Source: CAD feature listing. Evaluate the final solid. Frame: model axes, mm. Give positions to 0.01 mm unless a question says otherwise; leave off trailing zeros. Write each loop counter-clockwise with the first axis right and the second up, starting at its lowest first coordinate (ties: lowest second). Pieces come first, ordered by that corner, then holes. Notation, with made-up numbers: M 84,28.5 L 113,28.5 A30 ccw 113,55.5 Z; hole C 5.5,77 d10. An arc over 180 degrees is marked long. Use CSV: the item, a comma, the result in double quotes. Start each with the question number.
from build123d import *

# Parameters (mm, degrees)
SKETCH1_R           = 1.25
BOSS_EXTRUDE1_DEPTH = 5
FILLET1_R           = 20


with BuildPart() as part:
    # Sketch1 → Boss-Extrude1 (new body)
    with BuildSketch(Plane.XY):
        with BuildLine():
            Line((32, 5), (-32, 5))
            Line((-32, 5), (-32, 59.644660941))
            ThreePointArc((-32, 59.644660941), (-30.47759065, 67.298329588), (-26.142135624, 73.786796564))
            Line((-26.142135624, 73.786796564), (-14.142135624, 85.786796564))
            ThreePointArc((-14.142135624, 85.786796564), (0, 91.644660941), (14.142135624, 85.786796564))
            Line((14.142135624, 85.786796564), (26.142135624, 73.786796564))
            ThreePointArc((26.142135624, 73.786796564), (30.47759065, 67.298329588), (32, 59.644660941))
            Line((32, 59.644660941), (32, 5))
        make_face()
        with Locations((0, 85.644660941)):
            Circle(SKETCH1_R, mode=Mode.SUBTRACT)
        with Locations((-13.102089171, 78.341561643)):
            Circle(SKETCH1_R, mode=Mode.SUBTRACT)
        with Locations((-23.708690889, 67.734959925)):
            Circle(SKETCH1_R, mode=Mode.SUBTRACT)
        with Locations((-26, 52.910996131)):
            Circle(SKETCH1_R, mode=Mode.SUBTRACT)
        with Locations((-26, 36.198039027)):
            Circle(SKETCH1_R, mode=Mode.SUBTRACT)
        with Locations((-26, 21.198039027)):
            Circle(SKETCH1_R, mode=Mode.SUBTRACT)
        with Locations((0, 11)):
            Circle(SKETCH1_R, mode=Mode.SUBTRACT)
        with Locations((-15, 11)):
            Circle(SKETCH1_R, mode=Mode.SUBTRACT)
        with Locations(Location((13.102089171, 78.341561643, 0), (0, 0, 180))):
            Circle(SKETCH1_R, mode=Mode.SUBTRACT)
        with Locations(Location((23.708690889, 67.734959925, 0), (0, 0, 180))):
            Circle(SKETCH1_R, mode=Mode.SUBTRACT)
        with Locations(Location((26, 52.910996131, 0), (0, 0, 180))):
            Circle(SKETCH1_R, mode=Mode.SUBTRACT)
        with Locations(Location((26, 36.198039027, 0), (0, 0, 180))):
            Circle(SKETCH1_R, mode=Mode.SUBTRACT)
        with Locations(Location((26, 21.198039027, 0), (0, 0, 180))):
            Circle(SKETCH1_R, mode=Mode.SUBTRACT)
        with Locations(Location((15, 11, 0), (0, 0, 180))):
            Circle(SKETCH1_R, mode=Mode.SUBTRACT)
    extrude(amount=BOSS_EXTRUDE1_DEPTH)

    # Fillet1
    fillet1_edges = [part.edges().sort_by_distance(p)[0] for p in [
        (32, 5, 2.5),
        (-32, 5, 2.5),
    ]]
    fillet(fillet1_edges, radius=FILLET1_R)


solid = part.part
Item 1: Section C-C (z = 2.65). State how many separate pieces and enclosed holes the cut face has, plus the area to 3 significant figures.
Item 2: Material intervals for probe 1 along Y at (x, z) = (0, 1.35); probe 2 along Y at (x, z) = (26, 3); probe 3 along X at (y, z) = (86, 3.65), sorted ascending.
Item 3: Contact query for a flat-ended pin moving along its axis: pin 1 Ø2 at (x, y) = (-15, 11) entering from +Z. Output: stop coordinate, or through.
Item 4: Section B-B (y = 11). Return the cut outline in (x, z), plus the area to 3 significant figures.
Item 5: Section D-D (x = 19). Return the cut outline in (y, z) (3 decimals), plus the area to 3 significant figures.
Item 6: Pull-direction query (X, two-part tool) for faces 1 (the flat face through (-32, 42, 2)), 2 (the flat face through (32, 43, 2)), 3 (the flat face through (0, 49, 5)), 4 (the cylindrical face through (15.16, 9.76, 2.46)); classes: released by +X, released by -X, zero draft, split by the parting line, or undercut.
Item 7: Section A-A (x = 0). Return the cut outline in (y, z).
Output values:
1,separate pieces,"1"
1,enclosed holes,"14"
1,area,"4,710 mm2"
2,probe 1,"y = 5 to 9.75, 12.25 to 84.39, 86.89 to 91.64"
2,probe 2,"y = 10.72 to 19.95, 22.45 to 34.95, 37.45 to 51.66, 54.16 to 73.93"
2,probe 3,"x = -13.93 to -1.2, 1.2 to 13.93"
3,pin 1,"passes through"
4,outline,"M -26.28,0 L -16.25,0 L -16.25,5 L -26.28,5 Z; M -13.75,0 L -1.25,0 L -1.25,5 L -13.75,5 Z; M 1.25,0 L 13.75,0 L 13.75,5 L 1.25,5 Z; M 16.25,0 L 26.28,0 L 26.28,5 L 16.25,5 Z"
4,area,"225 mm2"
5,outline,"M 6.265,0 L 80.929,0 L 80.929,5 L 6.265,5 Z"
5,area,"373 mm2"
6,face 1,"released by -X"
6,face 2,"released by +X"
6,face 3,"zero draft"
6,face 4,"undercut"
7,outline,"M 5,0 L 9.75,0 L 9.75,5 L 5,5 Z; M 12.25,0 L 84.39,0 L 84.39,5 L 12.25,5 Z; M 86.89,0 L 91.64,0 L 91.64,5 L 86.89,5 Z"
